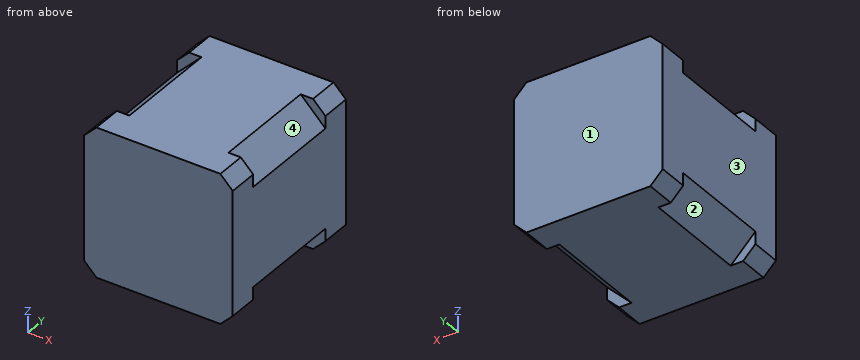
```python
from build123d import *

# Parameters (mm, degrees)
BOX013_W        = 42
BOX013_H        = 8.5
BOX013_DEPTH    = 42
CHAMFER001_SIZE = 3.5
BOX_W           = 42
BOX_H           = 30
BOX_DEPTH       = 42
CHAMFER002_SIZE = 7
BOX012_W        = 42
BOX012_H        = 8.5
BOX012_DEPTH    = 42
CHAMFER_SIZE    = 3.5


with BuildPart() as chamfer001:
    # Box013 → Box013 (new body)
    with BuildSketch(Plane(origin=(7, 43.5, 2.5), x_dir=(1, 0, 0), z_dir=(0, 0, 1))):
        with Locations((21, 4.25)):
            Rectangle(BOX013_W, BOX013_H)
    extrude(amount=BOX013_DEPTH)

    # Chamfer001
    chamfer001_edges = [chamfer001.edges().sort_by_distance(p)[0] for p in [
        (7, 47.75, 44.5),
        (7, 47.75, 2.5),
        (49, 47.75, 44.5),
        (49, 47.75, 2.5),
    ]]
    chamfer(chamfer001_edges, length=CHAMFER001_SIZE)


with BuildPart() as chamfer002:
    # Box → Box (new body)
    with BuildSketch(Plane(origin=(7, 13.5, 2.5), x_dir=(1, 0, 0), z_dir=(0, 0, 1))):
        with Locations((21, 15)):
            Rectangle(BOX_W, BOX_H)
    extrude(amount=BOX_DEPTH)

    # Chamfer002
    chamfer002_edges = [chamfer002.edges().sort_by_distance(p)[0] for p in [
        (7, 28.5, 44.5),
        (7, 28.5, 2.5),
        (49, 28.5, 44.5),
        (49, 28.5, 2.5),
    ]]
    chamfer(chamfer002_edges, length=CHAMFER002_SIZE)


with BuildPart() as do_not_print_nema17_dummy:
    # Box012 → Box012 (new body)
    with BuildSketch(Plane(origin=(7, 5, 2.5), x_dir=(1, 0, 0), z_dir=(0, 0, 1))):
        with Locations((21, 4.25)):
            Rectangle(BOX012_W, BOX012_H)
    extrude(amount=BOX012_DEPTH)

    # Chamfer
    chamfer_edges = [do_not_print_nema17_dummy.edges().sort_by_distance(p)[0] for p in [
        (7, 9.25, 44.5),
        (7, 9.25, 2.5),
        (49, 9.25, 44.5),
        (49, 9.25, 2.5),
    ]]
    chamfer(chamfer_edges, length=CHAMFER_SIZE)

    # Fusion: union Chamfer001, Chamfer002
    add(chamfer001.part)
    add(chamfer002.part)


solid = do_not_print_nema17_dummy.part
```
Read the model definition and answer for the solid it produces. Units are mm, in the model's axes. Face numbers are marked on the shaded views. Give positions to 0.01 mm unless a question says otherwise; leave off trailing zeros. Order: outer loops, then holes, each group sorted by start corner. A loop starts at its lowest first (then second) coordinate and runs counter-clockwise, first axis right, second up. Notation, with made-up numbers: (85.25, 26.5) -> (91.25, 26.5) arc R35 cw to (91.25, 61.5) -> close; hole circle Ø8 at (83, 81). An arc over 180 degrees is marked (long way). Write item = value, one per line.
1. A cutting plane is placed at A-A, the plane y = 30. Write down the section's boundary in (x, z).
Numbers:
outline = (7, 9.5) -> (14, 2.5) -> (42, 2.5) -> (49, 9.5) -> (49, 37.5) -> (42, 44.5) -> (14, 44.5) -> (7, 37.5) -> close
2. A cutting plane is placed at C-C, the plane x = 43. Write down the section's boundary in (y, z), and give its area (3 significant figures).
Numbers:
outline = (5, 2.5) -> (13.5, 2.5) -> (13.5, 3.5) -> (43.5, 3.5) -> (43.5, 2.5) -> (52, 2.5) -> (52, 44.5) -> (43.5, 44.5) -> (43.5, 43.5) -> (13.5, 43.5) -> (13.5, 44.5) -> (5, 44.5) -> close
area = 1,910 mm²
3. Straight lines are drawn through the part: line 1 along X through (y, z) = (29.5, 42); line 2 along Z through (x, y) = (10, 20); line 3 along Z through (x, y) = (9, 40.5). For each, find the intervals that lie inside material, in ascending order.
Numbers:
line_1 = 11.5 to 44.5
line_2 = 6.5 to 40.5
line_3 = 7.5 to 39.5
4. A cutting plane is placed at B-B, the plane z = 7.5. Write down the section's boundary in (x, y).
Numbers:
outline = (7, 5) -> (49, 5) -> (49, 13.5) -> (47, 13.5) -> (47, 43.5) -> (49, 43.5) -> (49, 52) -> (7, 52) -> (7, 43.5) -> (9, 43.5) -> (9, 13.5) -> (7, 13.5) -> close
5. Given pin 1 (4 mm diameter, centred on y = 21.5, z = 7, fed in from +X), flat-ended and moving along its own axis, determine where the tip first touches the part or whether it passes through.
Numbers:
pin_1 = 48.5
6. The mould has two halves that part along Y. Classify the marked faces 1, 2, 3 and 4: +Y half, -Y half, draft (parallel to the pull), parting line (faces both ways), or undercut.
Numbers:
face_1 = +Y half
face_2 = undercut
face_3 = draft
face_4 = undercut
